from build123d import *

# Parameters (mm, degrees)
F0_W      = 106.426
F0_H      = 66.294
F1_DEPTH  = 35.941
F2_W      = 12.7
F2_H      = 12.954
F3_DEPTH  = 12.192
F4_W      = 10.414
F4_H      = 9.652
F5_DEPTH  = 12.7
F6_W      = 10.414
F6_H      = 9.652
F7_DEPTH  = 12.7
F8_R      = 3.175
F9_DEPTH  = 1.27
F10_R     = 3.175
F11_DEPTH = 1.27


with BuildPart() as f1:
    # F0 (on Top) → F1 (new body, symmetric)
    with BuildSketch(Plane.XY):
        Rectangle(F0_W, F0_H)
    extrude(amount=F1_DEPTH, both=True)

    # F2 (on face) → F3 (join)
    with BuildSketch(Plane.XY.offset(35.941)):
        Polygon((50.673, 30.607), (-50.673, 30.607), (-50.673, -12.573), (-12.573, -12.573), (-12.573, -30.607), (31.877, -30.607), (31.877, -12.573), (50.673, -12.573), align=None)
        with Locations((-44.323, -24.13)):
            Rectangle(F2_W, F2_H)
        with Locations((44.323, -24.13)):
            Rectangle(F2_W, F2_H)
    extrude(amount=F3_DEPTH)

    # F4 (on face) → F5 (cut)
    with BuildSketch(Plane(origin=(-50.673, 0, 0), x_dir=(0, -1, 0), z_dir=(-1, 0, 0))):
        with Locations((24.13, 42.037)):
            Rectangle(F4_W, F4_H)
    extrude(amount=-F5_DEPTH, mode=Mode.SUBTRACT)

    # F6 (on face) → F7 (cut)
    with BuildSketch(Plane.YZ.offset(50.673)):
        with Locations((-24.13, 42.037)):
            Rectangle(F6_W, F6_H)
    extrude(amount=-F7_DEPTH, mode=Mode.SUBTRACT)

    # F8 (on face) → F9 (cut)
    with BuildSketch(Plane.XY.offset(48.133)):
        with Locations((-44.323, -24.13)):
            Circle(F8_R)
    extrude(amount=-F9_DEPTH, mode=Mode.SUBTRACT)

    # F10 (on face) → F11 (cut)
    with BuildSketch(Plane.XY.offset(48.133)):
        with Locations((44.323, -24.13)):
            Circle(F10_R)
    extrude(amount=-F11_DEPTH, mode=Mode.SUBTRACT)


solid = f1.part
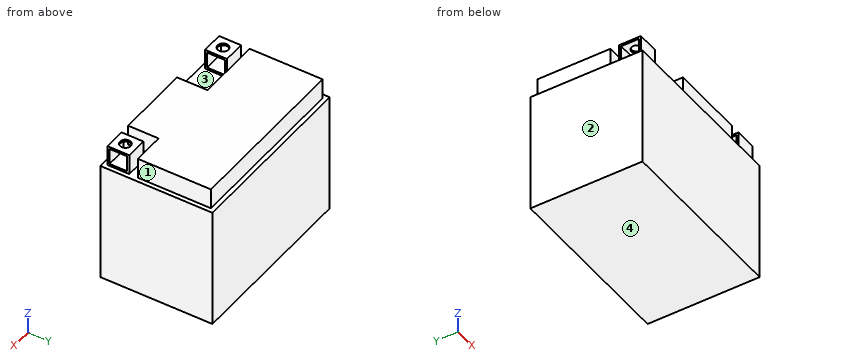
The listing builds one solid part. Answer for the finished solid, in the listing's coordinates (mm). Face numbers are marked on the shaded views. Round coordinates to 2 decimals unless told otherwise and drop trailing zeros. Write each loop counter-clockwise with the first axis right and the second up, starting at its lowest first coordinate (ties: lowest second). Pieces come first, ordered by that corner, then holes. Notation, with made-up numbers: M -7.5,-18.75 L 34.5,-18.75 A21 ccw 34.5,-7.75 Z; hole C 17,-38.5 d11. An arc over 180 degrees is marked long. Write each question's results on one line, items separated by ' | '. Start each with the question number.
Item 1: For a pull along X with two mould halves and no side action, classify the marked faces 1, 2, 3 and 4 as pulls with the +X half, pulls with the -X half, needs draft (parallel to the pull), parting line crosses it, or undercut.
Item 2: A cutting plane is placed at A-A on y = -24.13. State how many separate pieces and enclosed holes the cut face has, and give its area (3 significant figures).
Item 3: Flat-ended cylindrical pins translate along their axes: pin 1 Ø3.5 at (x, z) = (11, 43) entering from +Y; pin 2 Ø3.5 at (y, z) = (-24, 43) entering from -X; pin 3 Ø6 at (x, z) = (-41.5, 41.5) entering from -Y. Find the tip coordinate at first contact, or state that the pin passes through.
Item 4: Straight lines are drawn through the part: L1, parallel to X at y = -24, z = 47; L2, parallel to Z at x = 34, y = -17; L3, parallel to Y at x = -19, z = 41. For each, find the intervals that lie inside material, in ascending order. Write a range as [from, to].
Item 5: A cutting plane is placed at B-B on x = -29. Write down the section's boundary in (y, z), and give its area (3 significant figures).
Check sheet entries:
1) face 1: pulls with the +X half | face 2: pulls with the -X half | face 3: undercut | face 4: needs draft
2) separate pieces: 5 | enclosed holes: 0 | area: 8,240 mm²
3) pin 1: y = 30.61 | pin 2: x = -12.57 | pin 3: y = -30.61
4) L1: [-50.67, -47.5], [-41.15, -37.97], [-12.57, 31.88], [37.97, 41.15], [47.5, 50.67] | L2: [-35.94, 35.94] | L3: [-12.57, 30.61]
5) outline: M -33.15,-35.94 L 33.15,-35.94 L 33.15,35.94 L 30.61,35.94 L 30.61,48.13 L -12.57,48.13 L -12.57,35.94 L -33.15,35.94 Z | area: 5,290 mm²
